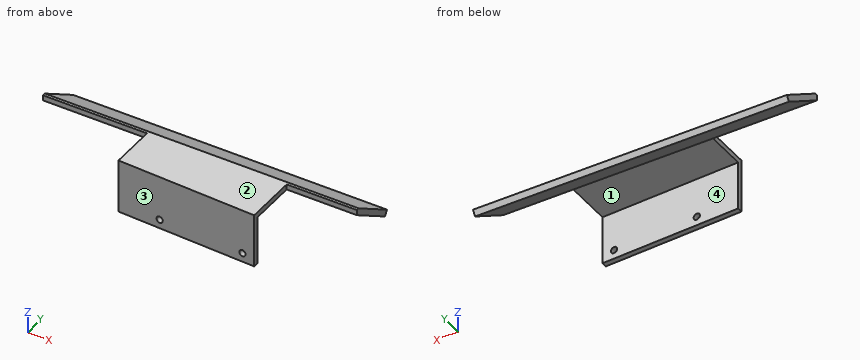
```python
from build123d import *

# Parameters (mm, degrees)
BOSS_EXTRUDE1_DEPTH     = 175
BOSS_EXTRUDE2_DEPTH     = 3
SKETCH3_W               = 175.182761709
SKETCH3_H               = 30
BOSS_EXTRUDE3_DEPTH     = 3
CUT_EXTRUDE2_DEPTH      = 181.792640115
CUT_EXTRUDE2_DEPTH_BACK = 181.792640115
CUT_EXTRUDE3_DEPTH      = 184.561872553
CUT_EXTRUDE3_DEPTH_BACK = 184.561872553
SKETCH6_R               = 1.8
CUT_EXTRUDE4_DEPTH      = 181.463142487
CUT_EXTRUDE4_DEPTH_BACK = 181.463142487
SKETCH7_W               = 17.123749229
SKETCH7_H               = 37.285884773


with BuildPart() as part:
    # Sketch1 → Boss-Extrude1 (new body)
    with BuildSketch(Plane(origin=(0, 0, 0), x_dir=(0, 0, -1), z_dir=(1, 0, 0))):
        Polygon((-8.588191211, -21.709603514), (-8.588191211, -3.209603514), (7.989641648, 22.272457974), (10.839609051, 20.418358247), (-5.588191211, -4.833085652), (-5.588191211, -21.709603514), align=None)
    extrude(amount=BOSS_EXTRUDE1_DEPTH)

    # Sketch2 → Boss-Extrude2 (add)
    with BuildSketch(Plane(origin=(0, 0, 5.588191211), x_dir=(-1, 0, 0), z_dir=(0, 0, -1))):
        Polygon((-175, -4.833085652), (-175, -35.833085652), (0, -27.833085652), (0, -4.833085652), align=None)
    extrude(amount=-BOSS_EXTRUDE2_DEPTH)

    # Sketch3 → Boss-Extrude3 (add)
    with BuildSketch(Plane(origin=(-1.269716182, -27.775041484, 0), x_dir=(0.9989567369115598, -0.045666593687385605, 0), z_dir=(-0.045666593687385605, -0.9989567369115598, 0))):
        with Locations((88.862423069, -6.411808789)):
            Rectangle(SKETCH3_W, SKETCH3_H)
    extrude(amount=-BOSS_EXTRUDE3_DEPTH)

    # Sketch5 → Cut-Extrude2 (cut, two sides: drawn at the far end of the back side and taken through both)
    with BuildSketch(Plane(origin=(0, 0, 5.588191211), x_dir=(-1, 0, 0), z_dir=(0, 0, -1)).offset(-CUT_EXTRUDE2_DEPTH_BACK)):
        Polygon((-153, -31.824238309), (-153, -4.833085652), (-175, -4.833085652), (-175, -32.829952595), align=None)
        Polygon((-153, -39.90576601), (-153, -31.824238309), (-175, -32.829952595), (-175, -4.833085652), (-195.370559552, -4.833085652), (-195.370559552, -39.90576601), align=None)
        Polygon((-0.136999781, -24.836215442), (-58, -27.481381166), (-58, -41.473834752), (0, -41.473834752), (0, -27.833085652), align=None)
        Polygon((0, -4.833085652), (-58, -4.833085652), (-58, -27.481381166), (-0.136999781, -24.836215442), (0, -27.833085652), align=None)
    extrude(amount=CUT_EXTRUDE2_DEPTH + CUT_EXTRUDE2_DEPTH_BACK, mode=Mode.SUBTRACT)

    # Sketch6 → Cut-Extrude3 (cut, two sides: drawn at the far end of the back side and taken through both)
    with BuildSketch(Plane(origin=(-1.132716401, -24.778171273, 0), x_dir=(0.9989567369115598, -0.045666593687385605, 0), z_dir=(0.045666593687385605, 0.9989567369115598, 0)).offset(-CUT_EXTRUDE3_DEPTH_BACK)):
        with Locations(Location((82.969275183, 16.411808789, 0), (0, 0, 180))):
            Circle(SKETCH6_R)
        with Locations((130.518881933, 16.411808789)):
            Circle(SKETCH6_R)
    extrude(amount=CUT_EXTRUDE3_DEPTH + CUT_EXTRUDE3_DEPTH_BACK, mode=Mode.SUBTRACT)

    # Sketch7 → Cut-Extrude4 (cut, two sides: drawn at the far end of the back side and taken through both)
    with BuildSketch(Plane(origin=(0, 0, 5.588191211), x_dir=(-1, 0, 0), z_dir=(0, 0, -1)).offset(-CUT_EXTRUDE4_DEPTH_BACK)):
        with Locations((-144.438125386, -23.476028039)):
            Rectangle(SKETCH7_W, SKETCH7_H)
    extrude(amount=CUT_EXTRUDE4_DEPTH + CUT_EXTRUDE4_DEPTH_BACK, mode=Mode.SUBTRACT)


solid = part.part
```
Here's how the part is built. I have some questions about the finished solid (model axes, mm). Face numbers are marked on the shaded views. Round coordinates to 2 decimals unless told otherwise and drop trailing zeros. Order: outer loops, then holes, each group sorted by start corner. A loop starts at its lowest first (then second) coordinate and runs counter-clockwise, first axis right, second up. Notation, with made-up numbers: M -26,-2 L 21,-2 A13 cw 21,20 Z; hole C 8,16.25 d1. An arc over 180 degrees is marked long. Answer in a Markdown table with one row per item.
Item 1: If I drill on L1, parallel to Z at x = 117, y = -21; L2, parallel to Y at x = 79.5, z = -7.5; L3, parallel to X at y = -16, z = 6, over which ranges is the centre line in solid material (lowest first)? Write a range as from..to.
A:
| item | result |
|---|---|
| L1 | z = 5.59..8.59 |
| L2 | y = -31.47..-28.46, 15.28..21.52 |
| L3 | x = 58..135.88 |
Item 2: Imagine slicing it at B-B, the plane x = 33. Write out the boundary of the cut face in (y, z).
A:
| item | result |
|---|---|
| outline | M -4.83,5.59 L 20.42,-10.84 L 22.27,-7.99 L -3.21,8.59 L -4.83,8.59 Z |
Item 3: I'm going to push flat-ended pins straight in: pin 1 (6 mm diameter, centred on x = 156.5, z = -15, fed in from +Y); pin 2 (0.9 mm diameter, centred on x = 16.5, z = 7, fed in from -Y); pin 3 (1 mm diameter, centred on x = 74.5, y = 1, fed in from +Z); pin 4 (1.5 mm diameter, centred on x = 89, y = -26, fed in from -Z). Where does each tip first touch, or does it pass through?
A:
| item | result |
|---|---|
| pin 1 | passes through |
| pin 2 | stops at y = -4.83 |
| pin 3 | stops at z = 6.17 |
| pin 4 | stops at z = 5.59 |
Item 4: Imagine slicing it at A-A, the plane z = -4.5. Write out the boundary of the cut face in (x, y).
A:
| item | result |
|---|---|
| outline | M 0,10.67 L 175,10.67 L 175,16.91 L 0,16.91 Z; M 58,-30.48 L 135.88,-34.04 L 135.88,-31.04 L 58,-27.48 Z |
Item 5: Imagine slicing it at D-D, the plane x = 105.5. Write out the boundary of the cut face in (y, z), and give its area (3 significant figures).
A:
| item | result |
|---|---|
| outline | M -32.66,-21.41 L -29.65,-21.41 L -29.65,5.59 L -4.83,5.59 L 20.42,-10.84 L 22.27,-7.99 L -3.21,8.59 L -32.66,8.59 Z |
| area | 270 mm2 |
Item 6: Thinking about a two-plate mould opening in Y: for the marked faces 1, 2, 3 and 4, which applies, +Y half, -Y half, draft (parallel to the pull), parting line (faces both ways), or undercut?
A:
| item | result |
|---|---|
| face 1 | undercut |
| face 2 | draft |
| face 3 | -Y half |
| face 4 | undercut |
Item 7: Imagine slicing it at C-C, the plane y = -6.5. Write out the boundary of the cut face in (x, z), and give its area (3 significant figures).
A:
| item | result |
|---|---|
| outline | M 58,5.59 L 135.88,5.59 L 135.88,8.59 L 58,8.59 Z |
| area | 234 mm2 |
